Geometry check sheet. Reference: the model listing, model coordinates, mm. A direction names the side the tool comes from. Round coordinates to 2 decimals unless told otherwise and drop trailing zeros. Order: outer loops, then holes, each group sorted by start corner. A loop starts at its lowest first (then second) coordinate and runs counter-clockwise, first axis right, second up. Notation, with made-up numbers: M 14,-4.75 L 48,-4.75 A18 cw 48,21.25 Z; hole C 9,-23 d10. An arc over 180 degrees is marked long. Answer as a JSON object with one key per item and string values. Group by question number.
```python
from build123d import *

# Parameters (mm, degrees)
CROQUIS1_W              = 230
CROQUIS1_H              = 230
CROQUIS1_R              = 2
SALIENTE_EXTRUIR1_DEPTH = 5
CROQUIS2_W              = 17.489873555
CROQUIS2_H              = 230
CROQUIS2_W_2            = 44.814479666
SALIENTE_EXTRUIR2_DEPTH = 5
CROQUIS3_W              = 91
CROQUIS3_H              = 3.3
CORTAR_EXTRUIR1_DEPTH   = 225
CROQUIS4_W              = 75.102886612
CROQUIS4_H              = 185
CORTAR_EXTRUIR2_DEPTH   = 256
CROQUIS5_R              = 2.6
CORTAR_EXTRUIR3_DEPTH   = 4
CROQUIS13_R             = 2
CORTAR_EXTRUIR5_DEPTH   = 88
CROQUIS14_R             = 3
CORTAR_EXTRUIR6_DEPTH   = 3
CROQUIS16_R             = 1.75
CORTAR_EXTRUIR7_DEPTH   = 3
CROQUIS18_W             = 230
CROQUIS18_H             = 10
SALIENTE_EXTRUIR4_DEPTH = 3


with BuildPart() as part:
    # Croquis1 → Saliente-Extruir1 (new body)
    with BuildSketch(Plane(origin=(0, 0, 0), x_dir=(1, 0, 0), z_dir=(0, 1, 0))):
        Rectangle(CROQUIS1_W, CROQUIS1_H)
        with Locations(Location((109.100078083, 109.100078083, 0), (0, 0, 270))):
            Circle(CROQUIS1_R, mode=Mode.SUBTRACT)
        with Locations(Location((-109.100078083, 109.100078083, 0), (0, 0, 270))):
            Circle(CROQUIS1_R, mode=Mode.SUBTRACT)
        with Locations(Location((-109.100078083, -109.100078083, 0), (0, 0, 270))):
            Circle(CROQUIS1_R, mode=Mode.SUBTRACT)
        with Locations(Location((109.100078083, -109.100078083, 0), (0, 0, 270))):
            Circle(CROQUIS1_R, mode=Mode.SUBTRACT)
    extrude(amount=SALIENTE_EXTRUIR1_DEPTH)

    # Croquis2 → Saliente-Extruir2 (add)
    with BuildSketch(Plane(origin=(0, 5, 0), x_dir=(1, 0, 0), z_dir=(0, 1, 0))):
        with Locations((-106.255063223, 0)):
            Rectangle(CROQUIS2_W, CROQUIS2_H)
        Rectangle(CROQUIS2_W_2, CROQUIS2_H)
        with Locations((106.255063223, 0)):
            Rectangle(CROQUIS2_W, CROQUIS2_H)
    extrude(amount=SALIENTE_EXTRUIR2_DEPTH)

    # Croquis3 → Cortar-Extruir1 (cut)
    with BuildSketch(Plane.XY.offset(115)):
        with Locations((-60.755063223, 6.65)):
            Rectangle(CROQUIS3_W, CROQUIS3_H)
        with Locations((60.755063223, 6.65)):
            Rectangle(CROQUIS3_W, CROQUIS3_H)
    extrude(amount=-CORTAR_EXTRUIR1_DEPTH, mode=Mode.SUBTRACT)

    # Croquis4 → Cortar-Extruir2 (cut)
    with BuildSketch(Plane(origin=(0, 5, 0), x_dir=(1, 0, 0), z_dir=(0, 1, 0))):
        with Locations((-59.448556694, -7.5)):
            Rectangle(CROQUIS4_W, CROQUIS4_H)
        with Locations((59.448556694, -7.5)):
            Rectangle(CROQUIS4_W, CROQUIS4_H)
    extrude(amount=-CORTAR_EXTRUIR2_DEPTH, mode=Mode.SUBTRACT)

    # Croquis5 → Cortar-Extruir3 (cut)
    with BuildSketch(Plane.XZ):
        with Locations(Location((-82, 105, 0), (0, 0, 270))):
            Circle(CROQUIS5_R)
        with Locations(Location((-36, 105, 0), (0, 0, 270))):
            Circle(CROQUIS5_R)
        with Locations(Location((-13, 105, 0), (0, 0, 270))):
            Circle(CROQUIS5_R)
        with Locations(Location((10, 105, 0), (0, 0, 270))):
            Circle(CROQUIS5_R)
        with Locations(Location((33, 105, 0), (0, 0, 270))):
            Circle(CROQUIS5_R)
        with Locations(Location((79, 105, 0), (0, 0, 270))):
            Circle(CROQUIS5_R)
        with Locations(Location((-13, 82, 0), (0, 0, 270))):
            Circle(CROQUIS5_R)
        with Locations(Location((10, 82, 0), (0, 0, 270))):
            Circle(CROQUIS5_R)
        with Locations(Location((102, 82, 0), (0, 0, 270))):
            Circle(CROQUIS5_R)
        with Locations(Location((-13, 13, 0), (0, 0, 270))):
            Circle(CROQUIS5_R)
        with Locations(Location((10, 13, 0), (0, 0, 270))):
            Circle(CROQUIS5_R)
        with Locations(Location((102, 13, 0), (0, 0, 270))):
            Circle(CROQUIS5_R)
        with Locations(Location((-13, -10, 0), (0, 0, 270))):
            Circle(CROQUIS5_R)
        with Locations(Location((10, -10, 0), (0, 0, 270))):
            Circle(CROQUIS5_R)
        with Locations(Location((102, -10, 0), (0, 0, 270))):
            Circle(CROQUIS5_R)
        with Locations(Location((-13, -79, 0), (0, 0, 270))):
            Circle(CROQUIS5_R)
        with Locations(Location((10, -79, 0), (0, 0, 270))):
            Circle(CROQUIS5_R)
        with Locations(Location((102, -79, 0), (0, 0, 270))):
            Circle(CROQUIS5_R)
        with Locations(Location((-82, -102, 0), (0, 0, 270))):
            Circle(CROQUIS5_R)
        with Locations(Location((-36, -102, 0), (0, 0, 270))):
            Circle(CROQUIS5_R)
        with Locations(Location((-13, -102, 0), (0, 0, 270))):
            Circle(CROQUIS5_R)
        with Locations(Location((10, -102, 0), (0, 0, 270))):
            Circle(CROQUIS5_R)
        with Locations(Location((33, -102, 0), (0, 0, 270))):
            Circle(CROQUIS5_R)
        with Locations(Location((79, -102, 0), (0, 0, 270))):
            Circle(CROQUIS5_R)
        with Locations(Location((-105, 82, 0), (0, 0, 270))):
            Circle(CROQUIS5_R)
        with Locations(Location((-105, 13, 0), (0, 0, 270))):
            Circle(CROQUIS5_R)
        with Locations(Location((-105, -10, 0), (0, 0, 270))):
            Circle(CROQUIS5_R)
        with Locations(Location((-105, -79, 0), (0, 0, 270))):
            Circle(CROQUIS5_R)
    extrude(amount=-CORTAR_EXTRUIR3_DEPTH, mode=Mode.SUBTRACT)

    # Croquis13 → Cortar-Extruir5 (cut)
    with BuildSketch(Plane.XZ.offset(-5)):
        with Locations(Location((-109.100078083, 109.100078083, 0), (0, 0, 90))):
            Circle(CROQUIS13_R)
        with Locations(Location((109.100078083, 109.100078083, 0), (0, 0, 90))):
            Circle(CROQUIS13_R)
        with Locations(Location((109.100078083, -109.100078083, 0), (0, 0, 90))):
            Circle(CROQUIS13_R)
        with Locations(Location((-109.100078083, -109.100078083, 0), (0, 0, 90))):
            Circle(CROQUIS13_R)
    extrude(amount=-CORTAR_EXTRUIR5_DEPTH, mode=Mode.SUBTRACT)

    # Croquis14 → Cortar-Extruir6 (cut)
    with BuildSketch(Plane(origin=(0, 0, 0), x_dir=(-1, 0, 0), z_dir=(0, -1, 0))):
        with Locations(Location((109.100078083, -109.100078083, 0), (0, 0, 90))):
            Circle(CROQUIS14_R)
        with Locations(Location((-109.100078083, -109.100078083, 0), (0, 0, 270))):
            Circle(CROQUIS14_R)
        with Locations(Location((-109.100078083, 109.100078083, 0), (0, 0, 90))):
            Circle(CROQUIS14_R)
        with Locations(Location((109.100078083, 109.100078083, 0), (0, 0, 270))):
            Circle(CROQUIS14_R)
    extrude(amount=-CORTAR_EXTRUIR6_DEPTH, mode=Mode.SUBTRACT)

    # Croquis16 → Cortar-Extruir7 (cut)
    with BuildSketch(Plane.XY.offset(115)):
        with Locations((0, 4.279276807)):
            Circle(CROQUIS16_R)
        with Locations((110.490700251, 4.279276807)):
            Circle(CROQUIS16_R)
        with Locations(Location((-110.490700251, 4.279276807, 0), (0, 0, 313.028420556))):
            Circle(CROQUIS16_R)
    extrude(amount=-CORTAR_EXTRUIR7_DEPTH, mode=Mode.SUBTRACT)

    # Croquis18 → Saliente-Extruir4 (add)
    with BuildSketch(Plane(origin=(0, 0, -115), x_dir=(-1, 0, 0), z_dir=(0, 0, -1))):
        with Locations((0, 5)):
            Rectangle(CROQUIS18_W, CROQUIS18_H)
    extrude(amount=-SALIENTE_EXTRUIR4_DEPTH)


solid = part.part
```
1) Thickness scan on line 1 along X through (y, z) = (2.75, 55); line 2 along X through (y, z) = (7.5, 5.5); line 3 along Y through (x, z) = (100, 101.5). Record the ranges inside material, lowest first. Write a range as [from, to].
2) Set-up check for faces 1 (the flat face through (-60, 3, 100)), 2 (the cylindrical face through (9, 2, 102.6)): record each of +Z, -Z, +X, -X, +Y, -Y from which the full face is reachable in a straight line by a thin tool's end or side.
3) Sectioned sample at A-A (z = 30). Record the boundary of the cut face in (x, y), then the cut area to 3 significant figures.
4) Sectioned sample at C-C (x = 18). Record the boundary of the cut face in (y, z), then the cut area to 3 significant figures.
5) Sectioned sample at B-B (x = 90). Record the boundary of the cut face in (y, z).
6) Go/stop test with a flat-tipped pin: P1, Ø3, axis at x = -13, z = 82, coming from the -Y side. Record where the tip stops, or that it passes through.
Final values:
{
 "1": {"line 1": "x = [-115, -97], [-21.9, 21.9], [97, 115]", "line 2": "x = [-115, -106.26], [-15.26, 15.26], [106.26, 115]", "line 3": "y = [0, 5], [8.3, 10]"},
 "2": {"face 1": "+Y, -Y", "face 2": "-Y"},
 "3": {"outline": "M -115,0 L -97,0 L -97,5 L -106.26,5 L -106.26,8.3 L -97.51,8.3 L -97.51,10 L -115,10 Z; M -22.41,8.3 L -15.26,8.3 L -15.26,5 L -21.9,5 L -21.9,0 L 21.9,0 L 21.9,5 L 15.26,5 L 15.26,8.3 L 22.41,8.3 L 22.41,10 L -22.41,10 Z; M 97,0 L 115,0 L 115,10 L 97.51,10 L 97.51,8.3 L 106.26,8.3 L 106.26,5 L 97,5 Z", "area": "693 mm^2"},
 "4": {"outline": "M 0,-115 L 10,-115 L 10,115 L 8.3,115 L 8.3,-110 L 5,-110 L 5,115 L 0,115 Z", "area": "1,560 mm^2"},
 "5": {"outline": "M 0,-115 L 10,-115 L 10,-112 L 5,-112 L 5,-85 L 0,-85 Z; M 0,100 L 5,100 L 5,115 L 0,115 Z"},
 "6": {"P1": "stops at y = 4"}
}
